The model under review builds one solid part; all positions refer to its coordinate system, in mm. Face numbers are marked on the shaded views. A direction names the side the tool comes from. Give positions to 0.01 mm unless a question says otherwise; leave off trailing zeros. Loops run counter-clockwise (first coordinate to the right, second up) from the corner with the lowest first, then second, coordinate; pieces in that order, holes last. Notation, with made-up numbers: M 22,23.25 L 28,23.25 A11 cw 28,37.25 Z; hole C -4,41 d10. An arc over 180 degrees is marked long. Write item = value, one per line. Start each with the question number.
1. For the marked faces 4, 5, 6 and 7, list the 3-axis set-ups (+Z, -Z, +X, -X, +Y, -Y) from which the entire face can be reached by the end or side of a thin tool; tool diameter is ignored.
2. We need section D-D on x = 83.5. Give the boundary of the cut face in (y, z), then the cut area to 3 significant figures.
3. We need section C-C on z = 153. Give the boundary of the cut face in (x, y).
4. For pin 1 (12.5 mm diameter, centred on y = -2, z = 178, fed in from -X); pin 2 (3 mm diameter, centred on x = -58.5, y = -13.5, fed in from +Z); pin 3 (22.5 mm diameter, centred on y = 2, z = 28, fed in from +X), all flat-tipped, find the tip position at first contact; note any pin that passes through.
5. Wall thickness on line 1 along Z through (x, y) = (21.75, -2); line 2 along X through (y, z) = (-6.5, 47); line 3 along Y through (x, z) = (4, 10): over which ranges is each line inside the solid? List them lowest first. Write a range as from..to.
6. We need section A-A on z = 28. Give the boundary of the cut face in (x, y).
7. Draft analysis for pull direction Y (two halves, no side actions). For the marked faces 1, 2 and 3, state which applies: pulls with the +Y half, pulls with the -Y half, needs draft (parallel to the pull), parting line crosses it, or undercut.
8. We need section B-B on x = -2. Give the boundary of the cut face in (y, z), then the cut area to 3 significant figures.
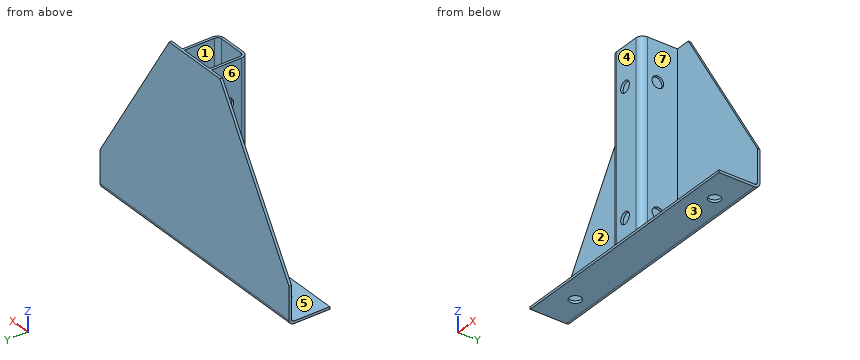
Autodesk Inventor part; units mm, degrees
ref_plane "YZ Plane" through (0, 0, 0) normal (1, 0, 0) x (0, 1, 0)
ref_plane "XZ Plane" through (0, 0, 0) normal (0, 1, 0) x (-1, 0, 0)
ref_plane "XY Plane" through (0, 0, 0) normal (0, 0, 1) x (1, 0, 0)
sketch "Sketch1" plane through (0, 0, 0) normal (0, 0, 1) x (1, 0, 0)
  line L0 (-152.5, -24.5) -> (152.5, -24.5)
  line L1 (152.5, -24.5) -> (152.5, 24.5)
  line L2 (152.5, 24.5) -> (-152.5, 24.5)
  line L3 (-152.5, 24.5) -> (-152.5, -24.5)
  point P0 (0, 24.5)
  point P1 (0, 0)
  point P2 (-152.5, 0)
  point P3 (0, -24.5)
  dimension "d0" = 305
  dimension "d1" = 49
extrude "Plate1" add sketch "Sketch1" along normal blind 3
sketch "Sketch2" plane through (152.5, 21.5, 0) normal (0, 1, 0) x (-1, 0, 0)
  line L0 (305, 0) -> (0, 0)
  line L1 (0, 0) -> (0, -225)
  line L2 (0, -225) -> (305, -225)
  line L3 (305, -225) -> (305, 0)
edge flange "Flange1" height 225 angle 90 thickness 3 bend radius 3 thickness toward (0, 1, 0) relief tear relief width 3 relief depth 1.5 edges at (0, 24.5, 0) wall of the first edge with corners at (-152.5, 21.5, 0) (152.5, 21.5, 0) (152.5, 21.5, 225) (-152.5, 21.5, 225)
bend "Bend1"
corner "Corner1"
chamfer "Corner Chamfer1" distance 111.5 distance2 180 1 edges at (152.5, 23, 225) measured on face at (-50.8333, 22.5, 225)
chamfer "Corner Chamfer2" distance 111.5 distance2 180 1 edges at (-152.5, 23, 225) measured on face at (-88, 22.5, 225)
sketch "Sketch4" plane through (0, 0, 3) normal (0, 0, 1) x (1, 0, 0)
  line L0 (152.5, -24.5) -> (-152.5, -24.5)
  line L1 (-112.5, 0) -> (112.5, 0)
  point P0 (0, 0)
  point P1 (0, 0)
  point P2 (0, -24.5)
  dimension "d26" = 225
  dimension "d27" = 24.5
hole "Hole1" at (-112.5, 0, 3) direction (0, 0, -1) diameter 14 end through all
pattern_linear "Rectangular Pattern1" count 2 spacing 225 along (1, 0, 0) of "Hole1"
sketch "Sketch3" plane through (-41, 21.5, 225) normal (0, 0, 1) x (1, 0, 0)
  line L0 (0, 0) -> (82, 0)
  line L1 (20.5, -41) -> (61.5, -41)
  line L2 (61.5, -41) -> (61.5, 0)
  line L3 (61.5, 0) -> (20.5, 0)
  line L4 (20.5, 0) -> (20.5, -41)
  line L5 (17.5, 0) -> (17.5, -44)
  line L6 (17.5, -44) -> (64.5, -44)
  line L7 (64.5, -44) -> (64.5, 0)
  point P0 (41, -21.5)
  point P1 (41, 0)
  dimension "d19" = 41
  dimension "d20" = 41
  dimension "d21" = 3
  dimension "d22" = 3
  dimension "d23" = 3
extrude "Extrusion1" add sketch "Sketch3" against normal up to next contours L0 L4 L1 L2 L7 L6 L5
fillet "Fillet1" radius 5 2 edges at (-20.5, -19.5, 114) (20.5, -19.5, 114)
fillet "Fillet1" radius 8 2 edges at (-23.5, -22.5, 114) (23.5, -22.5, 114)
hole "Hole2" at (23.5, -2, 28) direction (-1, 0, 0) diameter 14 depth 20 tip angle 118
pattern_linear "Rectangular Pattern2" count 2 spacing 150 along (0, 0, 1) of "Hole2"
pattern_circular "Circular Pattern1" count 3 over 180 about axis through (0, 0, -10) along (0, 0, -1) of "Hole2", "Rectangular Pattern2"
equation "\"d33\" = Thickness"
equation "\"d37\" = d26"
equation "\"d20\" = d19"
equation "\"d21\" = Thickness"
equation "\"d22\" = Thickness"
equation "\"d23\" = Thickness"
equation "\"d55\" = Thickness"
equation "\"d3\" = BendReliefWidth"
equation "\"d4\" = BendReliefDepth"
equation "\"d5\" = MinimumRemnant"
equation "\"d6\" = BendRadius"
equation "\"d9\" = BendRadius"
equation "\"d10\" = CornerReliefSize"
equation "\"d11\" = GapSize"
equation "\"d12\" = JacobiRadiusSize"
equation "\"BendRadius\" = Thickness"
equation "\"BendReliefWidth\" = Thickness"
equation "\"BendReliefDepth\" = 0.5 * Thickness"
equation "\"CornerReliefSize\" = 4 * Thickness"
equation "\"MinimumRemnant\" = 2 * Thickness"
equation "\"TransitionRadius\" = BendRadius"
equation "\"JacobiRadiusSize\" = BendRadius"
equation "\"GapSize\" = Thickness"
equation "\"d2\" = BendRadius"
properties part number "P2348-S1-Unistrut"
Final values:
q1.face_4 = +Z, +X, -X, -Y
q1.face_5 = +Z, -Y
q1.face_6 = +Z, -X, -Y
q1.face_7 = +Z, +X, -Y
q2.outline = M -24.5,0 L 18.5,0 A6 ccw 24.5,6 L 24.5,156.39 L 21.5,156.39 L 21.5,6 A3 cw 18.5,3 L -24.5,3 Z
q2.area = 601 mm²
q3.outline = M -85.6,21.5 L -23.5,21.5 L -23.5,-14.5 A8 ccw -15.5,-22.5 L 15.5,-22.5 A8 ccw 23.5,-14.5 L 23.5,21.5 L 85.6,21.5 L 85.6,24.5 L -85.6,24.5 Z; hole M -20.5,-14.5 A5 ccw -15.5,-19.5 L 15.5,-19.5 A5 ccw 20.5,-14.5 L 20.5,21.5 L -20.5,21.5 Z
q4.pin_1 = -23.5
q4.pin_2 = 3
q4.pin_3 = 23.5
q5.line_1 = 0..21, 35..171, 185..225
q5.line_2 = -23.5..-20.5, 20.5..23.5
q5.line_3 = -22.5..-19.5, 21.5..24.5
q6.outline = M -152.5,21.5 L -23.5,21.5 L -23.5,9 L -20.5,9 L -20.5,21.5 L 20.5,21.5 L 20.5,5 L 23.5,5 L 23.5,21.5 L 152.5,21.5 L 152.5,24.5 L -152.5,24.5 Z; M -23.5,-14.5 A8 ccw -15.5,-22.5 L -9,-22.5 L -9,-19.5 L -15.5,-19.5 A5 cw -20.5,-14.5 L -20.5,-5 L -23.5,-5 Z; M 5,-22.5 L 15.5,-22.5 A8 ccw 23.5,-14.5 L 23.5,-9 L 20.5,-9 L 20.5,-14.5 A5 cw 15.5,-19.5 L 5,-19.5 Z
q7.face_1 = undercut
q7.face_2 = pulls with the -Y half
q7.face_3 = needs draft
q8.outline = M -24.5,0 L 18.5,0 A6 ccw 24.5,6 L 24.5,225 L 21.5,225 L 21.5,6 A3 cw 18.5,3 L -19.5,3 L -19.5,21 L -22.5,21 L -22.5,3 L -24.5,3 Z; M -22.5,35 L -19.5,35 L -19.5,171 L -22.5,171 Z; M -22.5,185 L -19.5,185 L -19.5,225 L -22.5,225 Z
q8.area = 1,390 mm²
